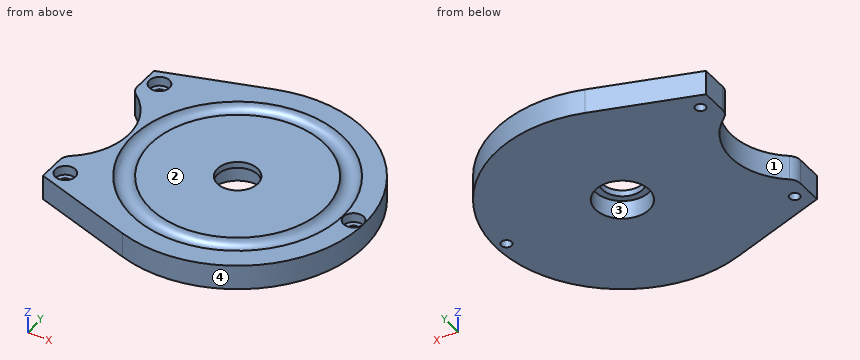
from build123d import *

# Parameters (mm, degrees)
F0_R            = 40.8
F1_DEPTH        = 8
F4_R            = 3.15
F8_DEPTH        = 8
F9_R            = 21
F10_DEPTH       = 8.001
F11_R           = 4
F13_D           = 3.3
F13_CBORE_D     = 6.5
F13_CBORE_DEPTH = 3


with BuildPart() as f1:
    # F0 (on Top) → F1 (new body)
    with BuildSketch(Plane.XY):
        Circle(F0_R)
    extrude(amount=F1_DEPTH)

    # F2 (on Right) → F3 (revolve, cut)
    with BuildSketch(Plane.YZ):
        Polygon((0, 8), (0, 0), (8.65, 0), (8.65, 6), (6.5, 6), (6.5, 8), align=None)
    revolve(axis=Axis((0, 0, 10.7360328796), (0, 0, 1)), mode=Mode.SUBTRACT)

    # F4 (on Right) → F5 (revolve, cut)
    with BuildSketch(Plane.YZ):
        with Locations((31, 9)):
            Circle(F4_R)
    revolve(axis=Axis((0, 0, 6.3867427816), (0, 0, 1)), mode=Mode.SUBTRACT)

    # F7 (on Top) → F8 (join, through all)
    with BuildSketch(Plane.XY):
        with BuildLine():
            Line((-45, 28.2782724184), (-45, -28.2782724184))
            Line((-45, -28.2782724184), (-12.6078933705, -38.8031058648))
            ThreePointArc((-12.6078933705, -38.8031058648), (-26.2059585661, -31.2711965814), (-36, -19.2))
            Line((-36, -19.2), (-36, 19.2))
            ThreePointArc((-36, 19.2), (-26.2059585661, 31.2711965814), (-12.6078933705, 38.8031058648))
            Line((-12.6078933705, 38.8031058648), (-45, 28.2782724184))
        make_face()
    extrude(amount=F8_DEPTH)

    # F9 (on face) → F10 (cut, through all)
    with BuildSketch(Plane.XY.offset(8)):
        with Locations((-56.25, 0)):
            Circle(F9_R)
    extrude(amount=-F10_DEPTH, mode=Mode.SUBTRACT)

    # F11
    f11_edges = [f1.edges().sort_by_distance(p)[0] for p in [
        (-45, 17.732386, 4),
        (-45, -17.732386, 4),
    ]]
    fillet(f11_edges, radius=F11_R)

    # F13 (through all)
    with Locations(Plane.XY.offset(8)):
        with Locations((-40.5, 24), (-40.5, -24), (37.5, 0)):
            CounterBoreHole(F13_D / 2, F13_CBORE_D / 2, F13_CBORE_DEPTH)


solid = f1.part
The model under review builds one solid part; all positions refer to its coordinate system, in mm. Face numbers are marked on the shaded views. Give positions to 0.01 mm unless a question says otherwise; leave off trailing zeros. Loops run counter-clockwise (first coordinate to the right, second up) from the corner with the lowest first, then second, coordinate; pieces in that order, holes last. Notation, with made-up numbers: (0, 27.5) -> (30, 27.5) arc R27 ccw to (30, 56.5) -> close; hole circle Ø5 at (-11, 25.5). An arc over 180 degrees is marked (long way). Answer as a JSON object with one key per item and string values. Group by question number.
Q1. Draft analysis for pull direction X (two halves, no side actions). For the marked faces 1, 2, 3 and 4, state which applies: pulls with the +X half, pulls with the -X half, needs draft (parallel to the pull), parting line crosses it, or undercut.
Q2. Insertion check: pin 1 (5 mm diameter, centred on x = 37.5, y = 0, fed in from +Z); pin 2 (2 mm diameter, centred on x = -40.5, y = 24, fed in from +Z); pin 3 (22.5 mm diameter, centred on x = 0, y = 0, fed in from -Z); pin 4 (4 mm diameter, centred on x = -26, z = 4.5, fed in from -Y). Each pin has a flat end and moves straight along its axis. Give the tip position at first contact, or say it passes through.
Q3. Wall thickness on line 1 along Y through (x, z) = (-40.5, 3.65); line 2 along Y through (x, z) = (0, 7.2); line 3 along Y through (x, z) = (4, 4): over which ranges is each line inside the solid? List them lowest first.
Q4. Take a section at B-B (x = 37.5). Write out the cut boundary in (y, z), plus the area to 3 significant figures.
Q5. Take a section at A-A (z = 7). Write out the cut boundary in (x, y).
Q6. Take a section at C-C (z = 2.75). Write out the cut boundary in (x, y), plus the area to 3 significant figures.
Q7. Take a section at D-D (x = -40.5). Write out the cut boundary in (y, z), plus the area to 3 significant figures.
Answer below:
{
 "1": {"face 1": "pulls with the -X half", "face 2": "needs draft", "face 3": "undercut", "face 4": "parting line crosses it"},
 "2": {"pin 1": "stops at z = 5", "pin 2": "passes through", "pin 3": "stops at z = 0", "pin 4": "stops at y = -35.1"},
 "3": {"line 1": "y = -29.74 to -25.65, -22.35 to -13.89, 13.89 to 22.35, 25.65 to 29.74", "line 2": "y = -40.8 to -33.59, -28.41 to -6.5, 6.5 to 28.41, 33.59 to 40.8", "line 3": "y = -40.6 to -7.67, 7.67 to 40.6"},
 "4": {"outline": "(-16.07, 0) -> (-1.65, 0) -> (-1.65, 5) -> (-3.25, 5) -> (-3.25, 8) -> (-16.07, 8) -> close; (1.65, 0) -> (16.07, 0) -> (16.07, 8) -> (3.25, 8) -> (3.25, 5) -> (1.65, 5) -> close", "area": "221 mm2"},
 "5": {"outline": "(-45, -28.28) -> (-12.61, -38.8) arc R40.8 ccw (long way) to (-12.61, 38.8) -> (-45, 28.28) -> (-45, 19.81) arc R4 ccw to (-43.44, 16.64) arc R21 cw to (-43.44, -16.64) arc R4 ccw to (-45, -19.81) -> close; circle Ø57.13 at (0, 0); hole circle Ø6.5 at (-40.5, -24); hole circle Ø6.5 at (-40.5, 24); hole circle Ø66.87 at (0, 0); hole circle Ø13 at (0, 0); hole circle Ø6.5 at (37.5, 0)"},
 "6": {"outline": "(-45, -28.28) -> (-12.61, -38.8) arc R40.8 ccw (long way) to (-12.61, 38.8) -> (-45, 28.28) -> (-45, 19.81) arc R4 ccw to (-43.44, 16.64) arc R21 cw to (-43.44, -16.64) arc R4 ccw to (-45, -19.81) -> close; hole circle Ø3.3 at (-40.5, -24); hole circle Ø3.3 at (-40.5, 24); hole circle Ø17.3 at (0, 0); hole circle Ø3.3 at (37.5, 0)", "area": "5,290 mm2"},
 "7": {"outline": "(-29.74, 0) -> (-25.65, 0) -> (-25.65, 5) -> (-27.25, 5) -> (-27.25, 8) -> (-29.74, 8) -> close; (-22.35, 0) -> (-13.89, 0) -> (-13.89, 8) -> (-20.75, 8) -> (-20.75, 5) -> (-22.35, 5) -> close; (13.89, 0) -> (22.35, 0) -> (22.35, 5) -> (20.75, 5) -> (20.75, 8) -> (13.89, 8) -> close; (25.65, 0) -> (29.74, 0) -> (29.74, 8) -> (27.25, 8) -> (27.25, 5) -> (25.65, 5) -> close", "area": "182 mm2"}
}
